Design review of the part built by this model. Coordinates are the model's own, in mm. A direction names the side the tool comes from. Round coordinates to 2 decimals unless told otherwise and drop trailing zeros. Loops run counter-clockwise (first coordinate to the right, second up) from the corner with the lowest first, then second, coordinate; pieces in that order, holes last. Notation, with made-up numbers: (51, -9) - (109, -9) arc R24 cw to (109, 3) - close; hole circle Ø3 at (28, 22). An arc over 180 degrees is marked (long way). Return JSON: item names as keys, results as strings. Group by question number.
(1) We need section A-A, the plane x = 23. Write out the cut boundary in (y, z).
(2) We need section D-D, the plane z = 5.75. Write out the cut boundary in (x, y).
(3) We need section B-B, the plane y = 5. Write out the cut boundary in (x, z).
(4) Wall thickness on L1, parallel to Y at x = 5, z = 1; L2, parallel to Z at x = 32, y = 2.5; L3, parallel to X at y = 3.25, z = 3.5: over which ranges is each line inside the solid? List them lowest first. Write a range as [from, to].
(5) Clearance check with flat-ended pins moving along their axes: pin 1 (1 mm diameter, centred on x = 19, z = 6, fed in from -Y); pin 2 (2 mm diameter, centred on y = 8.5, z = 5, fed in from +X); pin 3 (1 mm diameter, centred on x = 14, y = 8.5, fed in from +Z). State where each tip first meets the part, or that it passes through.
(6) For faces 4 (the cylindrical face through (19.8, 2.6, 5)), 5 (the cylindrical face through (45.715, 0.301, 1.521)), list the 3-axis set-ups (+Z, -Z, +X, -X, +Y, -Y) from which the entire face can be reached by the end or side of a thin tool; tool diameter is ignored.
(7) We need section C-C, the plane x = 5. Write out the cut boundary in (y, z), and give its area (3 significant figures).
(8) The part is to be moulded in two halves that separate along X. For faces 1 (the flat face through (23, 10, 1)), 2 (the cylindrical face through (3.415, 6.453, 1.479)), 3 (the cylindrical face through (0.301, 0.285, 1.521)), say which applies: pulls with the +X half, pulls with the -X half, needs draft (parallel to the pull), parting line crosses it, or undercut.
from build123d import *

# Parameters (mm, degrees)
SKETCH_W     = 46
SKETCH_H     = 10
SKETCH_R     = 2.15
PAD_DEPTH    = 3
SKETCH001_R  = 4
PAD001_DEPTH = 4
SKETCH002_R  = 2.15
POCKET_DEPTH = 7.001
FILLET_R     = 1
CHAMFER_SIZE = 0.4


with BuildPart() as part:
    # Sketch → Pad (new body)
    with BuildSketch(Plane.XY):
        with Locations((23, 5)):
            Rectangle(SKETCH_W, SKETCH_H)
        with Locations((5, 5)):
            Circle(SKETCH_R, mode=Mode.SUBTRACT)
        with Locations((41, 5)):
            Circle(SKETCH_R, mode=Mode.SUBTRACT)
        with Locations((23, 5)):
            Circle(SKETCH_R, mode=Mode.SUBTRACT)
    extrude(amount=PAD_DEPTH)

    # Sketch001 (on Face9 of Pad) → Pad001 (join)
    with BuildSketch(Plane.XY.offset(3)):
        with Locations((23, 5)):
            Circle(SKETCH001_R)
    extrude(amount=PAD001_DEPTH)

    # Sketch002 (on Face12 of Pad001) → Pocket (cut, through all)
    with BuildSketch(Plane.XY.offset(7)):
        with Locations((23, 5)):
            Circle(SKETCH002_R)
    extrude(amount=-POCKET_DEPTH, mode=Mode.SUBTRACT)

    # Fillet
    fillet_edges = [part.edges().sort_by_distance(p)[0] for p in [
        (0, 10, 1.5),
        (0, 0, 1.5),
        (46, 0, 1.5),
        (46, 10, 1.5),
    ]]
    fillet(fillet_edges, radius=FILLET_R)

    # Chamfer
    chamfer_edges = [part.edges().sort_by_distance(p)[0] for p in [
        (20.85, 5, 7),
    ]]
    chamfer(chamfer_edges, length=CHAMFER_SIZE)


solid = part.part
Solutions:
{
 "1": {"outline": "(0, 0) - (2.85, 0) - (2.85, 6.6) - (2.45, 7) - (1, 7) - (1, 3) - (0, 3) - close; (7.15, 0) - (10, 0) - (10, 3) - (9, 3) - (9, 7) - (7.55, 7) - (7.15, 6.6) - close"},
 "2": {"outline": "circle Ø8 at (23, 5); hole circle Ø4.3 at (23, 5)"},
 "3": {"outline": "(0, 0) - (2.85, 0) - (2.85, 3) - (0, 3) - close; (7.15, 0) - (20.85, 0) - (20.85, 6.6) - (20.45, 7) - (19, 7) - (19, 3) - (7.15, 3) - close; (25.15, 0) - (38.85, 0) - (38.85, 3) - (27, 3) - (27, 7) - (25.55, 7) - (25.15, 6.6) - close; (43.15, 0) - (46, 0) - (46, 3) - (43.15, 3) - close"},
 "4": {"L1": "[0, 2.85], [7.15, 10]", "L2": "[0, 3]", "L3": "[19.4, 21.75], [24.25, 26.6]"},
 "5": {"pin 1": "y = 3.06", "pin 2": "x = 26.12", "pin 3": "z = 3"},
 "6": {"face 4": "+Z", "face 5": "+Z, -Z, +X, -Y"},
 "7": {"outline": "(0, 0) - (2.85, 0) - (2.85, 3) - (0, 3) - close; (7.15, 0) - (10, 0) - (10, 3) - (7.15, 3) - close", "area": "17.1 mm^2"},
 "8": {"face 1": "needs draft", "face 2": "undercut", "face 3": "pulls with the -X half"}
}
